For this review, take the finished solid that the model builds, in its own axes (mm). A direction names the side the tool comes from. Give positions to 0.01 mm unless a question says otherwise; leave off trailing zeros. Order: outer loops, then holes, each group sorted by start corner. A loop starts at its lowest first (then second) coordinate and runs counter-clockwise, first axis right, second up. Notation, with made-up numbers: (-23, 17.5) - (-8, 17.5) arc R9 cw to (-8, 27.5) - close; hole circle Ø3 at (-27.5, -4). An arc over 180 degrees is marked (long way). Use a Markdown table: item, result. Add a question column.
1) Wall thickness on L1, parallel to X at y = -15, z = 14; L2, parallel to X at y = -2, z = 18; L3, parallel to Y at x = -13.5, z = 10: over which ranges is each line inside the solid? List them lowest first.
2) We need section B-B on x = 5. Write out the cut boundary in (y, z).
3) We need section C-C on x = 14. Write out the cut boundary in (y, z), then the cut area to 3 significant figures.
4) Machinability: for faces 1 (the face through (0, -5.567, 23)), 2 (the face through (6.754, -3.595, 25.939)), 3 (the face through (-12, -3, 28)), which of the approach directions +Z, -Z, +X, -X, +Y, -Y give a long, thin tool a straight path to every point of the face, cutting with its end or side? Answer none if there is none.
5) We need section A-A on z = 2. Write out the cut boundary in (x, y).
6) Clearance check with flat-ended pins moving along their axes: P1, Ø3, axis at x = -5, z = 27, coming from the -Y side; P2, Ø1.7, axis at y = -1.5, z = 7.5, coming from the -X side; P3, Ø3, axis at y = -3, z = 27, coming from the -X side; P4, Ø1.5, axis at x = 5, z = 27, coming from the +Y side. State where each tip first meets the part, or that it passes through.
7) Mouldability with a two-part tool opening along X and no side actions: class faces 4 (the face through (-17, -6, 0)), 5 (the face through (23.866, -15.377, 12.325)), 6 (the face through (-4.487, -3.595, 25.015)) as released by +X, released by -X, zero draft, split by the parting line, or undercut.
8) We need section D-D on x = -15.5. Write out the cut boundary in (y, z).
```python
from build123d import *

# Parameters (mm, degrees)
F1_DEPTH  = 25
F3_D      = 4.2
F5_D      = 4.2
F7_DEPTH  = 7
F9_DEPTH  = 25
F11_D     = 2.5
F13_DEPTH = 4


with BuildPart() as f1:
    # F0 (on Top) → F1 (new body)
    with BuildSketch(Plane.XY):
        Polygon((18.5, 0), (0, 0), (-18.5, 0), (-26.5, -13.856406), (-21.303848, -16.856406), (-14.785898, -5.566987), (0, -5.566987), (14.785898, -5.566987), (21.303848, -16.856406), (26.5, -13.856406), align=None)
    extrude(amount=F1_DEPTH)

    # F3 (through all)
    with Locations(Plane(origin=(-13.875, 8.010735, 0), x_dir=(-0.5, -0.866025, 0), z_dir=(-0.866025, 0.5, 0))):
        with Locations((17.75, 12.5)):
            Hole(F3_D / 2)

    # F5 (through all)
    with Locations(Plane(origin=(13.875, 8.010735, 0), x_dir=(-0.5, 0.866025, 0), z_dir=(0.866025, 0.5, 0))):
        with Locations((-17.75, 12.5)):
            Hole(F5_D / 2)

    # F6 (on face) → F7 (join)
    with BuildSketch(Plane.XY.offset(25)):
        Polygon((12, 0), (0, 0), (-12, 0), (-12, -5.566987), (12, -5.566987), align=None)
    extrude(amount=F7_DEPTH)

    # F8 (on face) → F9 (cut)
    with BuildSketch(Plane(origin=(0, 0, 0), x_dir=(-1, 0, 0), z_dir=(0, 1, 0))):
        with BuildLine():
            Line((7.996367, 0), (7.996367, 14.581786))
            ThreePointArc((7.996367, 14.581786), (0.121529, 22.821933), (-8, 14.824817))
            Line((-8, 14.824817), (-8.003633, 0))
            Line((-8.003633, 0), (7.996367, 0))
        make_face()
    extrude(amount=-F9_DEPTH, mode=Mode.SUBTRACT)

    # F11 (through all)
    with Locations(Plane(origin=(0, 0, 0), x_dir=(-1, 0, 0), z_dir=(0, 1, 0))):
        with Locations((5, 27), (-5, 27)):
            Hole(F11_D / 2)

    # F12 (on face) → F13 (cut)
    with BuildSketch(Plane.XZ.offset(5.566987)):
        Polygon((-5.614794, 24.714095), (-3.327745, 25.32462), (-2.712951, 27.610525), (-4.385206, 29.285905), (-6.672255, 28.67538), (-7.287049, 26.389475), align=None)
        Polygon((6.158304, 24.93562), (7.366958, 26.970931), (6.208654, 29.035311), (3.841696, 29.06438), (2.633042, 27.029069), (3.791346, 24.964689), align=None)
    extrude(amount=-F13_DEPTH, mode=Mode.SUBTRACT)


solid = f1.part
```
Checked values:
| question | item | result |
|---|---|---|
| 1 | L1 | -24.52 to -20.23, 20.23 to 24.52 |
| 1 | L2 | -19.65 to -7.34, 7.34 to 19.65 |
| 1 | L3 | -5.57 to 0 |
| 2 | outline | (-5.57, 21.07) - (0, 21.07) - (0, 25.75) - (-1.57, 25.75) - (-1.57, 24.95) - (-5.57, 24.95) - close; (-5.57, 29.05) - (-1.57, 29.05) - (-1.57, 28.25) - (0, 28.25) - (0, 32) - (-5.57, 32) - close |
| 3 | outline | (-5.57, 0) - (0, 0) - (0, 25) - (-5.57, 25) - close |
| 3 | area | 139 mm² |
| 4 | face 1 | +Z, -Z, -Y |
| 4 | face 2 | -Y |
| 4 | face 3 | +Z, -X, +Y, -Y |
| 5 | outline | (-26.5, -13.86) - (-21.3, -16.86) - (-14.79, -5.57) - (-8, -5.57) - (-8, 0) - (-18.5, 0) - close; (8, -5.57) - (14.79, -5.57) - (21.3, -16.86) - (26.5, -13.86) - (18.5, 0) - (8, 0) - close |
| 6 | P1 | y = -1.57 |
| 6 | P2 | x = -19.86 |
| 6 | P3 | x = -12 |
| 6 | P4 | through |
| 7 | face 4 | zero draft |
| 7 | face 5 | released by +X |
| 7 | face 6 | undercut |
| 8 | outline | (-6.8, 0) - (0, 0) - (0, 25) - (-6.8, 25) - close |
